```python
from build123d import *

# Parameters (mm, degrees)
BOSS_EXTRUDE1_DEPTH = 10.5
BOSS_EXTRUDE2_DEPTH = 2.5
SKETCH3_W           = 15
SKETCH3_H           = 62.5
BOSS_EXTRUDE3_DEPTH = 2.5
FILLET1_R           = 2.5
FILLET2_R           = 5


with BuildPart() as part:
    # Sketch1 → Boss-Extrude1 (new body)
    with BuildSketch(Plane.XY):
        Polygon((60, 60), (62.5, 60), (62.5, -2.5), (-2.5, -2.5), (-2.5, 60), (0, 60), (0, 0), (60, 0), align=None)
    extrude(amount=BOSS_EXTRUDE1_DEPTH)

    # Sketch2 → Boss-Extrude2 (add)
    with BuildSketch(Plane.XY.offset(10.5)):
        Polygon((52.5, 60), (62.5, 60), (62.5, -2.5), (-2.5, -2.5), (-2.5, 60), (7.5, 60), (7.5, 7.5), (52.5, 7.5), align=None)
    extrude(amount=BOSS_EXTRUDE2_DEPTH)

    # Sketch3 → Boss-Extrude3 (add)
    with BuildSketch(Plane(origin=(0, 0, 0), x_dir=(-1, 0, 0), z_dir=(0, 0, -1))):
        with Locations((-70, 28.75)):
            Rectangle(SKETCH3_W, SKETCH3_H)
        with Locations((10, 28.75)):
            Rectangle(SKETCH3_W, SKETCH3_H)
    extrude(amount=-BOSS_EXTRUDE3_DEPTH)

    # Fillet1
    fillet1_edges = [part.edges().sort_by_distance(p)[0] for p in [
        (0, 0, 5.25),
        (60, 0, 5.25),
        (60, 30, 10.5),
        (-2.5, 28.75, 13),
        (30, -2.5, 13),
        (62.5, 28.75, 13),
        (0, 30, 10.5),
        (62.5, 28.75, 2.5),
        (-2.5, 28.75, 2.5),
    ]]
    fillet(fillet1_edges, radius=FILLET1_R)

    # Fillet2
    fillet2_edges = [part.edges().sort_by_distance(p)[0] for p in [
        (7.5, 7.5, 11.75),
        (52.5, 7.5, 11.75),
        (-17.5, 60, 1.25),
        (-17.5, -2.5, 1.25),
        (77.5, -2.5, 1.25),
        (77.5, 60, 1.25),
        (52.5, 60, 11.75),
        (7.5, 60, 11.75),
    ]]
    fillet(fillet2_edges, radius=FILLET2_R)


solid = part.part
```
Check sheet for the modelled part. Datum: model origin and axes. Units: mm. A direction names the side the tool comes from. Round coordinates to 2 decimals unless told otherwise and drop trailing zeros. Loops run counter-clockwise (first coordinate to the right, second up) from the corner with the lowest first, then second, coordinate; pieces in that order, holes last. Notation, with made-up numbers: M -22,51.25 L 27,51.25 A22 ccw 27,59.25 Z; hole C 23,12 d6. An arc over 180 degrees is marked long. Answer as a JSON object with one key per item and string values.
1. Access from +Z, -Z, +X, -X, +Y, -Y to the whole of each face (thin tool, end or side, straight path). Record for faces 4 (the flat face through (-2.5, 28, 8)), 5 (the flat face through (62.5, 29, 8)), 6 (the flat face through (0, 32, 4)).
Reply:
{"face 4": "+Z, -X, +Y, -Y", "face 5": "+Z, +X, +Y, -Y", "face 6": "-Z, +Y"}
2. Section check D-D (x = 5). Record the boundary of the cut face in (y, z), plus the area to 3 significant figures.
Reply:
{"outline": "M -2.5,0 L 0,0 L 0,10.5 L 59.33,10.5 L 59.33,13 L 0,13 A2.5 ccw -2.5,10.5 Z", "area": "179 mm²"}
3. Section check B-B (z = 9.5). Record the boundary of the cut face in (x, y), plus the area to 3 significant figures.
Reply:
{"outline": "M -2.5,-2.5 L 62.5,-2.5 L 62.5,60 L 59.5,60 L 59.5,1 A2.5 cw 57.5,0 L 2.5,0 A2.5 cw 0.5,1 L 0.5,60 L -2.5,60 Z", "area": "524 mm²"}
4. Scan lines: line 1 (X direction, y = 4.5, z = 1); line 2 (X direction, y = 20, z = 8); line 3 (Y direction, x = 7, z = 8.75). Record each from-to range of solid material in increasing order.
Reply:
{"line 1": "x = -17.5 to 0, 60 to 77.5", "line 2": "x = -2.5 to 0, 60 to 62.5", "line 3": "y = -2.5 to 0"}
5. Mould release check, pull along X, two halves, no side actions. Record for faces 1 (the cylindrical face through (0.752, 0.713, 5.324)), 2 (the cylindrical face through (76.07, 58.5, 1.27)), 3 (the flat face through (62, 29, 0)): pulls with the +X half, pulls with the -X half, needs draft (parallel to the pull), parting line crosses it, or undercut.
Reply:
{"face 1": "undercut", "face 2": "pulls with the +X half", "face 3": "needs draft"}
6. Section check A-A (y = 53). Record the boundary of the cut face in (x, z).
Reply:
{"outline": "M -17.5,0 L 0,0 L 0,8 A2.5 cw 2.5,10.5 L 7.5,10.5 L 7.5,13 L 0,13 A2.5 ccw -2.5,10.5 L -2.5,5 A2.5 cw -5,2.5 L -17.5,2.5 Z; M 52.5,10.5 L 57.5,10.5 A2.5 cw 60,8 L 60,0 L 77.5,0 L 77.5,2.5 L 65,2.5 A2.5 cw 62.5,5 L 62.5,10.5 A2.5 ccw 60,13 L 52.5,13 Z"}
7. Section check C-C (x = 17). Record the boundary of the cut face in (y, z), plus the area to 3 significant figures.
Reply:
{"outline": "M -2.5,0 L 0,0 L 0,10.5 L 7.5,10.5 L 7.5,13 L 0,13 A2.5 ccw -2.5,10.5 Z", "area": "49.9 mm²"}
8. Gauge pin test, flat ends, axial feed: P1, Ø16.5, axis at x = 27, y = 16.5, coming from the -Z side; P2, Ø0.8, axis at y = 29.5, z = 11.5, coming from the +X side; P3, Ø1, axis at y = 4.5, z = 4.5, coming from the -X side; P4, Ø3, axis at x = 25, z = 11.5, coming from the +Y side. Record the tip position at first contact, or that the pin passes through.
Reply:
{"P1": "passes through", "P2": "stops at x = 62.43", "P3": "stops at x = -2.71", "P4": "stops at y = 7.5"}
